Design review of the part shown in the three views and the two pictorial views. Dimensions are in mm from the part's minimum x, y and z. Round coordinates to 2 decimals unless told otherwise and drop trailing zeros. Loops run counter-clockwise (first coordinate to the right, second up) from the corner with the lowest first, then second, coordinate; pieces in that order, holes last. Notation, with made-up numbers: (23, 29) -> (55, 29) arc R26 cw to (55, 55) -> close; hole circle Ø1 at (88.25, 79). An arc over 180 degrees is marked (long way). One line per question, with ' | ' between items. Start each with the question number.
1. Consider section B-B (x = 86.5). Write out the cut boundary in (y, z) (3 decimals), and give its area (3 significant figures).
2. Consider section C-C (z = 97). Write out the cut boundary in (x, y) (3 decimals), and give its area (3 significant figures).
3. For pin 1 Ø1 at (y, z) = (1, 68.5) entering from +X; pin 2 Ø1.6 at (x, y) = (260, 1) entering from -Z, all flat-tipped, find the tip position at first contact; note any pin that passes through.
4. Consider section A-A (y = 1.1). Write out the cut boundary in (x, z) (3 decimals), and give its area (3 significant figures).
5. Wall thickness on line 1 along Z through (x, y) = (300, 1.6); line 2 along X through (y, z) = (1.8, 56); line 3 along X through (y, z) = (2.3, 32.5): over which ranges is each line inside the solid? List them lowest first.
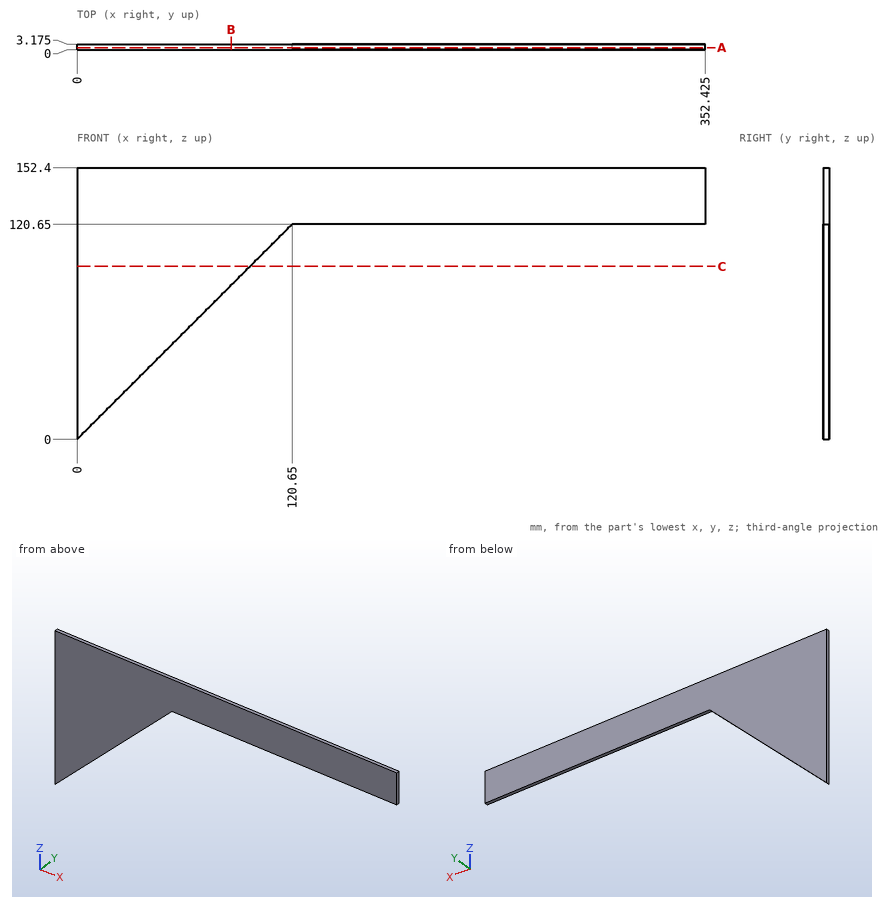
Answer block:
1) outline: (0, 86.5) -> (3.175, 86.5) -> (3.175, 152.4) -> (0, 152.4) -> close | area: 209 mm2
2) outline: (0, 0) -> (97, 0) -> (97, 3.175) -> (0, 3.175) -> close | area: 308 mm2
3) pin 1: stops at x = 69 | pin 2: stops at z = 120.65
4) outline: (0, 0) -> (120.65, 120.65) -> (352.425, 120.65) -> (352.425, 152.4) -> (0, 152.4) -> close | area: 18,500 mm2
5) line 1: z = 120.65 to 152.4 | line 2: x = 0 to 56 | line 3: x = 0 to 32.5
